Geometry check sheet. Reference: the model listing, model coordinates, mm. Face numbers are marked on the shaded views. Round coordinates to 2 decimals unless told otherwise and drop trailing zeros. Order: outer loops, then holes, each group sorted by start corner. A loop starts at its lowest first (then second) coordinate and runs counter-clockwise, first axis right, second up. Notation, with made-up numbers: (-12.75, 37.25) -> (2.25, 37.25) arc R10 ccw to (2.25, 41.25) -> close; hole circle Ø1 at (2, 36.5). An arc over 180 degrees is marked (long way). Use a Markdown table: item, result. Add a question column.
Item 1: Mould release check, pull along Y, two halves, no side actions. Record for the marked faces 1 and 2: pulls with the +Y half, pulls with the -Y half, needs draft (parallel to the pull), parting line crosses it, or undercut.
Item 2: Sectioned sample at B-B, the plane z = 1.05. Record the cut outline in (x, y).
Item 3: Material ranges on probe 1 along X at (y, z) = (-0.5, 0.55); probe 2 along Y at (x, z) = (0, 0.95); probe 3 along Z at (x, y) = (3.5, 1.5), recorded low to high. Write a range as [from, to].
Item 4: Sectioned sample at A-A, the plane z = 1.7. Record the cut outline in (x, y).
Item 5: Gauge pin test, flat ends, axial feed: pin 1 Ø1 at (y, z) = (-2.5, 0.5) entering from -X; pin 2 Ø4.5 at (x, y) = (0, 0) entering from -Z; pin 3 Ø1.5 at (x, z) = (3.5, 0.5) entering from +Y (3 decimals). Record the tip position at first contact, or that the pin passes through.
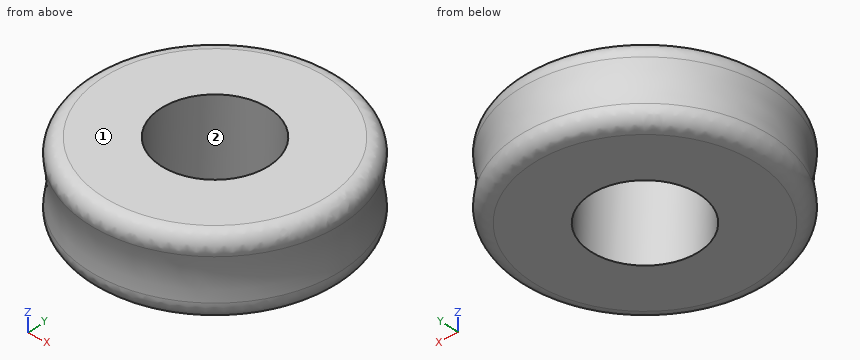
from build123d import *

# Parameters (mm, degrees)
SKETCH1_R           = 4.4323
SKETCH1_R_2         = 1.8161
BOSS_EXTRUDE1_DEPTH = 2.6162
FILLET1_R           = 0.5


with BuildPart() as part:
    # Sketch1 → Boss-Extrude1 (new body)
    with BuildSketch(Plane.XY):
        Circle(SKETCH1_R)
        Circle(SKETCH1_R_2, mode=Mode.SUBTRACT)
    extrude(amount=BOSS_EXTRUDE1_DEPTH)

    # Sketch2 → Cut-Revolve1 (revolve, cut)
    with BuildSketch(Plane(origin=(0, 0, 0), x_dir=(0, 0, -1), z_dir=(1, 0, 0)), mode=Mode.PRIVATE) as cut_revolve1_sk:
        with BuildLine():
            Line((-2.6162, 4.4323), (0, 4.4323))
            ThreePointArc((0, 4.4323), (-1.3081, 4.178663256), (-2.6162, 4.4323))
        make_face()
    revolve(cut_revolve1_sk.sketch.rotate(Axis((0, 0, 2.6162), (0, 0, -1)), 90), axis=Axis((0, 0, 2.6162), (0, 0, -1)), mode=Mode.SUBTRACT)

    # Fillet1
    fillet1_edges = [part.edges().sort_by_distance(p)[0] for p in [
        (-4.4323, 0, 2.6162),
        (-4.4323, 0, 0),
    ]]
    fillet(fillet1_edges, radius=FILLET1_R)


solid = part.part
Found:
| question | item | result |
|---|---|---|
| 1 | face 1 | needs draft |
| 1 | face 2 | undercut |
| 2 | outline | circle Ø8.38 at (0, 0); hole circle Ø3.63 at (0, 0) |
| 3 | probe 1 | x = [-4.23, -1.75], [1.75, 4.23] |
| 3 | probe 2 | y = [-4.2, -1.82], [1.82, 4.2] |
| 3 | probe 3 | z = [0, 2.61] |
| 4 | outline | circle Ø8.4 at (0, 0); hole circle Ø3.63 at (0, 0) |
| 5 | pin 1 | stops at x = -3.76 |
| 5 | pin 2 | stops at z = 0 |
| 5 | pin 3 | stops at y = 3.255 |
